Here's how the part is built. I have some questions about the finished solid (model axes, mm). A direction names the side the tool comes from. Round coordinates to 2 decimals unless told otherwise and drop trailing zeros. Loops run counter-clockwise (first coordinate to the right, second up) from the corner with the lowest first, then second, coordinate; pieces in that order, holes last. Notation, with made-up numbers: M -31,76.25 L 28,76.25 A7 ccw 28,83.25 Z; hole C -23.75,34 d9. An arc over 180 degrees is marked long. Use a Markdown table: item, result.
```python
from build123d import *

# Parameters (mm, degrees)
F0_W         = 76.2
F0_H         = 101.6
F1_DEPTH     = 25.4
F3_D         = 6.3754
F4_W         = 32.6189571008
F4_H         = 28.2830937386
F5_DEPTH     = 30.48
F6_T1_DEPTH  = 28.2830937386
F6_T6_DEPTH  = 32.6189571008
F6_S7_R      = 3.1877
F6_T8_DEPTH  = 18
F6_T13_DEPTH = 40.9830937386
F6_T17_DEPTH = 45.3189571008
F6_T20_DEPTH = 53.6830937386
F6_T22_DEPTH = 58.0189571008


# Not quite as in the source:
# - a fillet or chamfer that OpenCascade refuses, or shapes differently, is made with other operations: its cross-section is extruded or revolved along the edge and cut away or added


with BuildPart() as f1:
    # F0 (on Right) → F1 (new body)
    with BuildSketch(Plane.YZ):
        Rectangle(F0_W, F0_H)
    extrude(amount=F1_DEPTH)

    # F3 (through all)
    with Locations(Plane(origin=(0, 0, 0), x_dir=(0, -1, 0), z_dir=(-1, 0, 0))):
        with Locations((-31.3961266285, 0), (-9.7019366858, 29.8594908165), (25.4, 18.4541802113), (25.4, -18.4541802113), (-9.7019366858, -29.8594908165)):
            Hole(F3_D / 2)

    # F4 (on face) → F5 (join)
    with BuildSketch(Plane.YZ.offset(25.4)):
        with Locations((-21.7905214496, -36.6584531307)):
            Rectangle(F4_W, F4_H)
    extrude(amount=F5_DEPTH)

    # F6: fillet of radius 5.08 on 6 edges, made by hand

    # F6_s2 → F6_t1 (join)
    with BuildSketch(Plane.XY.offset(-50.8)):
        with BuildLine():
            ThreePointArc((25.4, -0.4010428992), (26.8878975516, -3.9931453476), (30.48, -5.4810428992))
            Line((30.48, -5.4810428992), (25.4, -5.4810428992))
            Line((25.4, -5.4810428992), (25.4, -0.4010428992))
        make_face()
    extrude(amount=F6_T1_DEPTH)


with BuildPart() as f6_tool4:
    # F6_s5 → F6_t6 (new body)
    with BuildSketch(Plane.XZ.offset(5.4810428992)):
        with BuildLine():
            ThreePointArc((25.4, -17.4369062614), (26.8878975516, -21.0290087099), (30.48, -22.5169062614))
            Line((30.48, -22.5169062614), (25.4, -22.5169062614))
            Line((25.4, -22.5169062614), (25.4, -17.4369062614))
        make_face()
    extrude(amount=F6_T6_DEPTH)

    # F6_s7 → F6_t8 (cut, symmetric)
    with BuildSketch(Plane.YZ.offset(27.9)):
        with Locations((-25.4, -18.4541802113)):
            Circle(F6_S7_R)
    extrude(amount=F6_T8_DEPTH, both=True, mode=Mode.SUBTRACT)


with BuildPart() as f1_1:
    add(f1.part)

    # F6_t3: union F6_tool4
    add(f6_tool4.part)


with BuildPart() as f6_tool11:
    # F6_s12 → F6_t13 (new body)
    with BuildSketch(Plane.XY.offset(-50.8)):
        with BuildLine():
            ThreePointArc((25.4, -0.4010428992), (26.8878975516, -3.9931453476), (30.48, -5.4810428992))
            Line((30.48, -5.4810428992), (25.4, -5.4810428992))
            Line((25.4, -5.4810428992), (25.4, -0.4010428992))
        make_face()
    extrude(amount=F6_T13_DEPTH)

    split(bisect_by=Plane.XY.offset(-22.5169062614), keep=Keep.TOP)


with BuildPart() as f6_tool15:
    # F6_s16 → F6_t17 (new body)
    with BuildSketch(Plane.XZ.offset(-7.2189571008)):
        with BuildLine():
            ThreePointArc((25.4, -17.4369062614), (26.8878975516, -21.0290087099), (30.48, -22.5169062614))
            Line((30.48, -22.5169062614), (25.4, -22.5169062614))
            Line((25.4, -22.5169062614), (25.4, -17.4369062614))
        make_face()
    extrude(amount=F6_T17_DEPTH)

    split(bisect_by=Plane.XZ.offset(5.4810428992), keep=Keep.BOTTOM)


with BuildPart() as f6_tool11_1:
    add(f6_tool11.part)

    # F6_t19: intersect F6_tool15
    add(f6_tool15.part, mode=Mode.INTERSECT)


with BuildPart() as f1_2:
    add(f1_1.part)

    # F6_t9: union F6_tool11
    add(f6_tool11_1.part)

    # F6_s21 → F6_t20 (cut)
    with BuildSketch(Plane.XY.offset(-63.5)):
        with BuildLine():
            ThreePointArc((50.8, -5.4810428992), (54.3921024484, -6.9689404508), (55.88, -10.5610428992))
            Line((55.88, -10.5610428992), (55.88, -5.4810428992))
            Line((55.88, -5.4810428992), (50.8, -5.4810428992))
        make_face()
        with BuildLine():
            ThreePointArc((55.88, -33.02), (54.3921024484, -36.6121024484), (50.8, -38.1))
            Line((50.8, -38.1), (55.88, -38.1))
            Line((55.88, -38.1), (55.88, -33.02))
        make_face()
    extrude(amount=F6_T20_DEPTH, mode=Mode.SUBTRACT)

    # F6_s23 → F6_t22 (cut)
    with BuildSketch(Plane.XZ.offset(-7.2189571008)):
        with BuildLine():
            ThreePointArc((55.88, -45.72), (54.3921024484, -49.3121024484), (50.8, -50.8))
            Line((50.8, -50.8), (55.88, -50.8))
            Line((55.88, -50.8), (55.88, -45.72))
        make_face()
        with BuildLine():
            ThreePointArc((55.88, -27.5969062614), (54.3921024484, -24.004803813), (50.8, -22.5169062614))
            Line((50.8, -22.5169062614), (55.88, -22.5169062614))
            Line((55.88, -22.5169062614), (55.88, -27.5969062614))
        make_face()
    extrude(amount=F6_T22_DEPTH, mode=Mode.SUBTRACT)


solid = f1_2.part
```
Q1. For faces 1 (the flat face through (40, -5.481, -37)), 2 (the flat face through (25.4, -1, 12)), 3 (the flat face through (20, -38.1, -11)), which set-ups out of +Z, -Z, +X, -X, +Y, -Y let a thin tool reach every point of the face, with its end or its side?
Return value:
| item | result |
|---|---|
| face 1 | +Z, -Z, +X, +Y |
| face 2 | +Z, +X, +Y |
| face 3 | +Z, -Z, +X, -X, -Y |
Q2. Imagine slicing it at C-C, the plane x = 24. Please give me the cut outline in (y, z), then the cut area to 3 significant figures.
Return value:
| item | result |
|---|---|
| outline | M -38.1,-50.8 L 38.1,-50.8 L 38.1,50.8 L -38.1,50.8 Z; hole C -25.4,-18.45 d6.38; hole C -25.4,18.45 d6.38; hole C 9.7,-29.86 d6.38; hole C 9.7,29.86 d6.38; hole C 31.4,0 d6.38 |
| area | 7,580 mm^2 |
Q3. I need wall thicknesses on line 1 (Z direction, x = 13, y = -25); line 2 (Z direction, x = 6, y = 9); line 3 (X direction, y = -4, z = 46.5). Which ranges of each line are inside material? Lowest first, please. Write a range as from..to.
Return value:
| item | result |
|---|---|
| line 1 | z = -50.8..-21.62, -15.29..15.29, 21.62..50.8 |
| line 2 | z = -50.8..-32.97, -26.75..26.75, 32.97..50.8 |
| line 3 | x = 0..25.4 |
Q4. Imagine slicing it at B-B, the plane y = -25.4. Please give me the cut outline in (x, z).
Return value:
| item | result |
|---|---|
| outline | M 0,-50.8 L 50.8,-50.8 A5.08 ccw 55.88,-45.72 L 55.88,-27.6 A5.08 ccw 50.8,-22.52 L 30.48,-22.52 A5.08 cw 27.63,-21.64 L 0,-21.64 Z; M 0,-15.27 L 25.4,-15.27 L 25.4,15.27 L 0,15.27 Z; M 0,21.64 L 25.4,21.64 L 25.4,50.8 L 0,50.8 Z |
Q5. Imagine slicing it at A-A, the plane z = 0. Please give me the cut outline in (x, y), then the cut area to 3 significant figures.
Return value:
| item | result |
|---|---|
| outline | M 0,-38.1 L 25.4,-38.1 L 25.4,28.21 L 0,28.21 Z; M 0,34.58 L 25.4,34.58 L 25.4,38.1 L 0,38.1 Z |
| area | 1,770 mm^2 |
Q6. Imagine slicing it at D-D, the plane z = -25.5. Please give me the cut outline in (x, y), then the cut area to 3 significant figures.
Return value:
| item | result |
|---|---|
| outline | M 0,-38.1 L 50.8,-38.1 A5.08 ccw 55.43,-35.12 L 55.43,-8.46 A5.08 ccw 50.8,-5.48 L 30.48,-5.48 A5.08 cw 25.4,-0.4 L 25.4,38.1 L 0,38.1 Z |
| area | 2,910 mm^2 |
Q7. Will these pins go through, and if not, where does the flat tip stop? P1, Ø5, axis at y = -0.5, z = -19, coming from the +X side; P2, Ø1, axis at y = 0.5, z = -13.5, coming from the -X side; P3, Ø4, axis at x = 41, z = -36.5, coming from the +Y side; P4, Ø10, axis at x = 45, y = -19, coming from the +Z side.
Return value:
| item | result |
|---|---|
| P1 | stops at x = 26.02 |
| P2 | stops at x = 0 |
| P3 | stops at y = -5.48 |
| P4 | stops at z = -22.52 |
Q8. We'd pull the mould along Z, two halves only. Please class faces 4 (the flat face through (41, -22, -22.517)), 5 (the flat face through (20, -8, -50.8)), 6 (the cylindrical face through (12.88, 34.34, -1.22)): pulls with the +Z half, pulls with the -Z half, needs draft (parallel to the pull), parting line crosses it, or undercut.
Return value:
| item | result |
|---|---|
| face 4 | pulls with the +Z half |
| face 5 | pulls with the -Z half |
| face 6 | undercut |
